```python
from build123d import *

# Parameters (mm, degrees)
SKETCH1_W               = 200
SKETCH1_H               = 100
BOSS_EXTRUDE1_DEPTH     = 2.6
FILLET1_R               = 10
SKETCH8_R               = 1.65
CUT_EXTRUDE4_DEPTH      = 2.6
LPATTERN1_COUNT         = 7
LPATTERN1_PITCH         = 6.35
MIRROR1_COPY_1_SKETCH_R = 1.65
MIRROR1_COPY_1_DEPTH    = 2.6
MIRROR1_COPY_2_SKETCH_R = 1.65
MIRROR1_COPY_2_DEPTH    = 2.6
MIRROR1_COPY_3_SKETCH_R = 1.65
MIRROR1_COPY_3_DEPTH    = 2.6
MIRROR1_COPY_4_SKETCH_R = 1.65
MIRROR1_COPY_4_DEPTH    = 2.6
MIRROR1_COPY_5_SKETCH_R = 1.65
MIRROR1_COPY_5_DEPTH    = 2.6
MIRROR1_COPY_6_SKETCH_R = 1.65
MIRROR1_COPY_6_DEPTH    = 2.6
SKETCH6_R               = 1.5
CUT_EXTRUDE6_DEPTH      = 2.6
MIRROR6_COPY_1_SKETCH_R = 1.5
MIRROR6_COPY_1_DEPTH    = 2.6
SKETCH13_R              = 4.980627928
CUT_EXTRUDE7_DEPTH      = 2.6
MIRROR8_COPY_1_SKETCH_R = 4.980627928
MIRROR8_COPY_1_DEPTH    = 2.6
SKETCH15_R              = 10
CUT_EXTRUDE8_DEPTH      = 2.6


with BuildPart() as part:
    # Sketch1 → Boss-Extrude1 (new body)
    with BuildSketch(Plane(origin=(0, 0, 0), x_dir=(1, 0, 0), z_dir=(0, 1, 0))):
        with Locations((100, -50)):
            Rectangle(SKETCH1_W, SKETCH1_H)
    extrude(amount=BOSS_EXTRUDE1_DEPTH)

    # Fillet1
    fillet1_edges = [part.edges().sort_by_distance(p)[0] for p in [
        (0, 1.3, 0),
        (200, 1.3, 0),
        (200, 1.3, 100),
        (0, 1.3, 100),
    ]]
    fillet(fillet1_edges, radius=FILLET1_R)

    # Sketch8 → Cut-Extrude4 (cut)
    with BuildSketch(Plane.XZ):
        with Locations(Location((192, 60.85, 0), (0, 0, 270))):
            Circle(SKETCH8_R)
        with Locations(Location((192, 39.15, 0), (0, 0, 270))):
            Circle(SKETCH8_R)
    cut_extrude4 = extrude(amount=-CUT_EXTRUDE4_DEPTH, mode=Mode.SUBTRACT)

    # LPattern1: Cut-Extrude4 ×7
    with Locations(*[(-i * LPATTERN1_PITCH, 0, 0) for i in range(1, LPATTERN1_COUNT)]):
        add(cut_extrude4, mode=Mode.SUBTRACT)

    # Mirror1: Cut-Extrude4 across plane
    add(cut_extrude4.mirror(Plane(origin=(100, 0, 0), x_dir=(0, 0, 1), z_dir=(1, 0, 0))), mode=Mode.SUBTRACT)

    # Mirror1 copy 1 sketch → Mirror1 copy 1 (cut)
    with BuildSketch(Plane(origin=(206.35, 0, 0), x_dir=(-1, 0, 0), z_dir=(0, -1, 0))):
        with Locations((192, -60.85)):
            Circle(MIRROR1_COPY_1_SKETCH_R)
        with Locations((192, -39.15)):
            Circle(MIRROR1_COPY_1_SKETCH_R)
    extrude(amount=-MIRROR1_COPY_1_DEPTH, mode=Mode.SUBTRACT)

    # Mirror1 copy 2 sketch → Mirror1 copy 2 (cut)
    with BuildSketch(Plane(origin=(212.7, 0, 0), x_dir=(-1, 0, 0), z_dir=(0, -1, 0))):
        with Locations((192, -60.85)):
            Circle(MIRROR1_COPY_2_SKETCH_R)
        with Locations((192, -39.15)):
            Circle(MIRROR1_COPY_2_SKETCH_R)
    extrude(amount=-MIRROR1_COPY_2_DEPTH, mode=Mode.SUBTRACT)

    # Mirror1 copy 3 sketch → Mirror1 copy 3 (cut)
    with BuildSketch(Plane(origin=(219.05, 0, 0), x_dir=(-1, 0, 0), z_dir=(0, -1, 0))):
        with Locations((192, -60.85)):
            Circle(MIRROR1_COPY_3_SKETCH_R)
        with Locations((192, -39.15)):
            Circle(MIRROR1_COPY_3_SKETCH_R)
    extrude(amount=-MIRROR1_COPY_3_DEPTH, mode=Mode.SUBTRACT)

    # Mirror1 copy 4 sketch → Mirror1 copy 4 (cut)
    with BuildSketch(Plane(origin=(225.4, 0, 0), x_dir=(-1, 0, 0), z_dir=(0, -1, 0))):
        with Locations((192, -60.85)):
            Circle(MIRROR1_COPY_4_SKETCH_R)
        with Locations((192, -39.15)):
            Circle(MIRROR1_COPY_4_SKETCH_R)
    extrude(amount=-MIRROR1_COPY_4_DEPTH, mode=Mode.SUBTRACT)

    # Mirror1 copy 5 sketch → Mirror1 copy 5 (cut)
    with BuildSketch(Plane(origin=(231.75, 0, 0), x_dir=(-1, 0, 0), z_dir=(0, -1, 0))):
        with Locations((192, -60.85)):
            Circle(MIRROR1_COPY_5_SKETCH_R)
        with Locations((192, -39.15)):
            Circle(MIRROR1_COPY_5_SKETCH_R)
    extrude(amount=-MIRROR1_COPY_5_DEPTH, mode=Mode.SUBTRACT)

    # Mirror1 copy 6 sketch → Mirror1 copy 6 (cut)
    with BuildSketch(Plane(origin=(238.1, 0, 0), x_dir=(-1, 0, 0), z_dir=(0, -1, 0))):
        with Locations((192, -60.85)):
            Circle(MIRROR1_COPY_6_SKETCH_R)
        with Locations((192, -39.15)):
            Circle(MIRROR1_COPY_6_SKETCH_R)
    extrude(amount=-MIRROR1_COPY_6_DEPTH, mode=Mode.SUBTRACT)

    # Sketch6 → Cut-Extrude6 (cut)
    with BuildSketch(Plane.XZ):
        with Locations(Location((190, 10, 0), (0, 0, 270))):
            Circle(SKETCH6_R)
    cut_extrude6 = extrude(amount=-CUT_EXTRUDE6_DEPTH, mode=Mode.SUBTRACT)

    # Mirror5: Cut-Extrude6 across plane
    add(cut_extrude6.mirror(Plane(origin=(100, 0, 0), x_dir=(0, 0, 1), z_dir=(1, 0, 0))), mode=Mode.SUBTRACT)

    # Mirror6: Cut-Extrude6 across plane
    add(cut_extrude6.mirror(Plane.XY.offset(50)), mode=Mode.SUBTRACT)

    # Mirror6 copy 1 sketch → Mirror6 copy 1 (cut)
    with BuildSketch(Plane(origin=(200, 0, 100), x_dir=(-1, 0, 0), z_dir=(0, -1, 0))):
        with Locations(Location((190, 10, 0), (0, 0, 270))):
            Circle(MIRROR6_COPY_1_SKETCH_R)
    extrude(amount=-MIRROR6_COPY_1_DEPTH, mode=Mode.SUBTRACT)

    # Sketch13 → Cut-Extrude7 (cut)
    with BuildSketch(Plane(origin=(0, 2.6, 0), x_dir=(1, 0, 0), z_dir=(0, 1, 0))):
        with Locations(Location((74, -80, 0), (0, 0, 270))):
            Circle(SKETCH13_R)
    cut_extrude7 = extrude(amount=-CUT_EXTRUDE7_DEPTH, mode=Mode.SUBTRACT)

    # Mirror7: Cut-Extrude7 across plane
    add(cut_extrude7.mirror(Plane.XY.offset(50)), mode=Mode.SUBTRACT)

    # Mirror8: Cut-Extrude7 across plane
    add(cut_extrude7.mirror(Plane(origin=(100, 0, 0), x_dir=(0, 0, 1), z_dir=(1, 0, 0))), mode=Mode.SUBTRACT)

    # Mirror8 copy 1 sketch → Mirror8 copy 1 (cut)
    with BuildSketch(Plane(origin=(200, 2.6, 100), x_dir=(-1, 0, 0), z_dir=(0, 1, 0))):
        with Locations(Location((74, -80, 0), (0, 0, 270))):
            Circle(MIRROR8_COPY_1_SKETCH_R)
    extrude(amount=-MIRROR8_COPY_1_DEPTH, mode=Mode.SUBTRACT)

    # Sketch15 → Cut-Extrude8 (cut)
    with BuildSketch(Plane.XZ):
        with Locations(Location((63.571852265, 49.722041857, 0), (0, 0, 270))):
            Circle(SKETCH15_R)
    cut_extrude8 = extrude(amount=-CUT_EXTRUDE8_DEPTH, mode=Mode.SUBTRACT)

    # Mirror9: Cut-Extrude8 across plane
    add(cut_extrude8.mirror(Plane(origin=(100, 0, 0), x_dir=(0, 0, 1), z_dir=(1, 0, 0))), mode=Mode.SUBTRACT)


solid = part.part
```
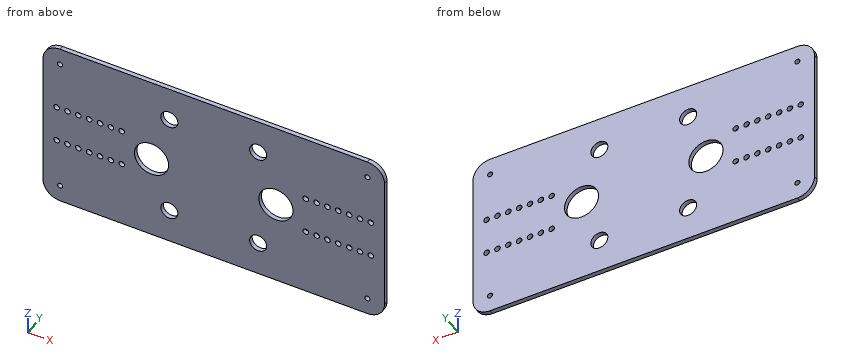
Input: part model. Units: mm. Frame: model coordinates. Round coordinates to 2 decimals unless told otherwise and drop trailing zeros. Loops run counter-clockwise (first coordinate to the right, second up) from the corner with the lowest first, then second, coordinate; pieces in that order, holes last. Notation, with made-up numbers: (13, 43.5) - (44, 43.5) arc R21 ccw to (44, 56.5) - close; hole circle Ø1 at (41.25, 80.25). An arc over 180 degrees is marked (long way). One line per item, written item: value. Start each with the question number.
(1) Section B-B, the plane z = 54.5. Return loops of the section in (x, y), plus the area to 3 significant figures.
(2) Section C-C, the plane y = 1.8. Count the separate pieces of the cut face and the enclosed holes in it, plus the area to 3 significant figures.
(3) Section A-A, the plane x = 134. Return loops of the section in (y, z), plus the area to 3 significant figures.
(4) Contact query for a flat-ended pin moving along its axis: P1, Ø4.5, axis at x = 20.7, z = 39.15, coming from the +Y side. Output: stop coordinate, or through.
(5) Ray query, line 1 (Z direction, x = 190, y = 0.9); line 2 (X direction, y = 0.85, z = 90); line 3 (Z direction, x = 39.75, y = 2.05). Return the intervals inside material, ascending. Write a range as [from, to].
Results below:
1. outline: (0, 0) - (54.79, 0) - (54.79, 2.6) - (0, 2.6) - close; (72.36, 0) - (127.64, 0) - (127.64, 2.6) - (72.36, 2.6) - close; (145.21, 0) - (200, 0) - (200, 2.6) - (145.21, 2.6) - close
1. area: 429 mm^2
2. separate pieces: 1
2. enclosed holes: 38
2. area: 18,700 mm^2
3. outline: (0, 0) - (2.6, 0) - (2.6, 40.02) - (0, 40.02) - close; (0, 59.42) - (2.6, 59.42) - (2.6, 100) - (0, 100) - close
3. area: 210 mm^2
4. P1: y = 2.6
5. line 1: [0, 8.5], [11.5, 88.5], [91.5, 100]
5. line 2: [0, 8.5], [11.5, 188.5], [191.5, 200]
5. line 3: [0, 37.5], [40.8, 59.2], [62.5, 100]
